Build history of the part. All positions in model axes, mm. Face numbers are marked on the shaded views. A direction names the side the tool comes from. Round coordinates to 2 decimals unless told otherwise and drop trailing zeros. Write each loop counter-clockwise with the first axis right and the second up, starting at its lowest first coordinate (ties: lowest second). Pieces come first, ordered by that corner, then holes. Notation, with made-up numbers: M 41,40 L 53,40 A19 cw 53,66 Z; hole C 29,-21 d7. An arc over 180 degrees is marked long. Write item = value, one per line. Start each with the question number.
Q1. Tool access for the marked faces 1, 2 and 3: list every direction of +Z, -Z, +X, -X, +Y, -Y with a clear straight run to the whole face (end or side of a thin tool).
Q2. Band-saw the part on A-A on y = 11. Write the cut outline in (x, z), plus the area to 3 significant figures.
Q3. Band-saw the part on D-D on y = -8. Write the cut outline in (x, z).
Q4. Band-saw the part on B-B on x = -0.5. Write the cut outline in (y, z).
Q5. Drop flat-ended pins along their axis: P1, Ø19, axis at x = -7.5, y = 5, coming from the +Z side; P2, Ø7.5, axis at y = -8, z = 26.5, coming from the -X side; P3, Ø10, axis at y = 5.5, z = 23, coming from the -X side; P4, Ø8, axis at x = -3, z = 28.5, coming from the -Y side. Give the stop position or say it passes through.
Q6. Band-saw the part on C-C on z = 23. Write the cut outline in (x, y).
Q7. Probe L1, parallel to Y at x = -6.5, z = 20; L2, parallel to Z at x = -15, y = 9; L3, parallel to X at y = -5, z = 31. List the from-to ranges inside material, lowest first.
Q8. Pull direction Y, two halves, no side cores. Call the marked faces 4, 5 and 6: released by +Y, released by -Y, zero draft, split by the parting line, or undercut.
```python
from build123d import *

# Parameters (mm, degrees)
F0_W     = 60.96
F0_H     = 38.1
F1_DEPTH = 10.16
F2_W     = 19.05
F2_H     = 38.1
F3_DEPTH = 25.4
F4_W     = 23.755038
F4_H     = 38.1
F5_DEPTH = 11.43
F6_W     = 23.755038
F6_H     = 17.78
F7_DEPTH = 11.43


with BuildPart() as f1:
    # F0 (on Top) → F1 (new body)
    with BuildSketch(Plane.XY):
        Rectangle(F0_W, F0_H)
    extrude(amount=F1_DEPTH)

    # F2 (on face) → F3 (join)
    with BuildSketch(Plane.XY.offset(10.16)):
        with Locations((20.955, 0)):
            Rectangle(F2_W, F2_H)
    extrude(amount=F3_DEPTH)

    # F4 (on face) → F5 (join)
    with BuildSketch(Plane.XY.offset(10.16)):
        with Locations((-0.447519, 0)):
            Rectangle(F4_W, F4_H)
    extrude(amount=F5_DEPTH)

    # F6 (on face) → F7 (cut, through all)
    with BuildSketch(Plane.XY.offset(21.59)):
        with Locations((-0.447519, 0)):
            Rectangle(F6_W, F6_H)
    extrude(amount=-F7_DEPTH, mode=Mode.SUBTRACT)


solid = f1.part
```
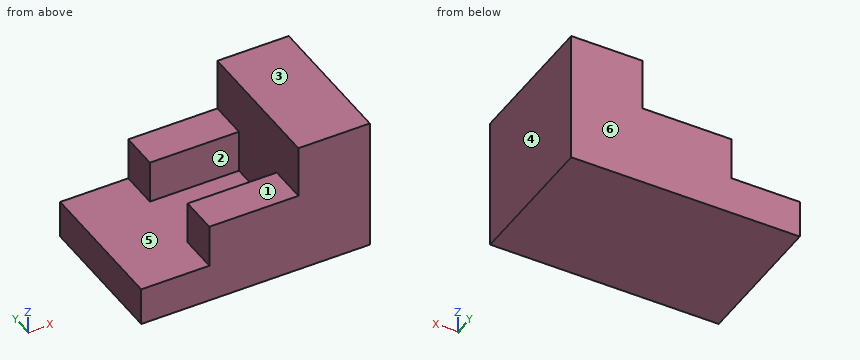
Conclusion:
q1.face_1 = +Z, -X, +Y, -Y
q1.face_2 = +Z, -X
q1.face_3 = +Z, +X, -X, +Y, -Y
q2.outline = M -30.48,0 L 30.48,0 L 30.48,35.56 L 11.43,35.56 L 11.43,21.59 L -12.33,21.59 L -12.33,10.16 L -30.48,10.16 Z
q2.area = 1,370 mm^2
q3.outline = M -30.48,0 L 30.48,0 L 30.48,35.56 L 11.43,35.56 L 11.43,10.16 L -30.48,10.16 Z
q4.outline = M -19.05,0 L 19.05,0 L 19.05,21.59 L 8.89,21.59 L 8.89,10.16 L -8.89,10.16 L -8.89,21.59 L -19.05,21.59 Z
q5.P1 = 21.59
q5.P2 = 11.43
q5.P3 = -12.33
q5.P4 = through
q6.outline = M 11.43,-19.05 L 30.48,-19.05 L 30.48,19.05 L 11.43,19.05 Z
q7.L1 = -19.05 to -8.89, 8.89 to 19.05
q7.L2 = 0 to 10.16
q7.L3 = 11.43 to 30.48
q8.face_4 = zero draft
q8.face_5 = undercut
q8.face_6 = released by +Y
